from build123d import *

# Parameters (mm, degrees)
BOSS_EXTRUDE1_DEPTH = 8
FILLET1_R           = 0.5
FILLET2_R           = 0.25


with BuildPart() as part:
    # Sketch1 → Boss-Extrude1 (new body)
    with BuildSketch(Plane.XY):
        Polygon((14, 0), (-14, 0), (-14, 7), (-7, 10), (7, 10), (14, 7), align=None)
        Polygon((12.5, 1.5), (-12.5, 1.5), (-12.5, 6.010905763), (-6.692113447, 8.5), (6.692113447, 8.5), (12.5, 6.010905763), align=None, mode=Mode.SUBTRACT)
    extrude(amount=BOSS_EXTRUDE1_DEPTH)

    # Fillet1
    fillet1_edges = [part.edges().sort_by_distance(p)[0] for p in [
        (14, 0, 4),
        (-14, 0, 4),
        (-14, 7, 4),
        (-7, 10, 4),
        (7, 10, 4),
        (14, 7, 4),
        (12.5, 1.5, 4),
        (12.5, 6.010905763, 4),
        (6.692113447, 8.5, 4),
        (-6.692113447, 8.5, 4),
        (-12.5, 6.010905763, 4),
        (-12.5, 1.5, 4),
    ]]
    fillet(fillet1_edges, radius=FILLET1_R)

    # Fillet2
    fillet2_edges = [part.edges().sort_by_distance(p)[0] for p in [
        (0, 1.5, 0),
        (0, 1.5, 8),
        (12.5, 3.840603842, 0),
        (12.5, 3.840603842, 8),
        (9.491701947, 7.300176357, 0),
        (9.491701947, 7.300176357, 8),
        (0, 8.5, 0),
        (0, 8.5, 8),
        (-9.491701947, 7.300176357, 0),
        (-9.491701947, 7.300176357, 8),
        (-12.5, 3.840603842, 0),
        (-12.5, 3.840603842, 8),
        (10.395645224, 8.544723476, 0),
        (10.395645224, 8.544723476, 8),
        (14, 3.585150961, 0),
        (0, 0, 0),
        (-14, 3.585150961, 0),
        (-10.395645224, 8.544723476, 0),
        (0, 10, 0),
        (6.997904085, 9.989788861, 0),
        (-6.997904085, 9.989788861, 0),
        (-13.917420546, 6.945547425, 0),
        (-13.853553391, 0.146446609, 0),
        (13.853553391, 0.146446609, 0),
        (13.917420546, 6.945547425, 0),
        (14, 3.585150961, 8),
        (0, 10, 8),
        (-10.395645224, 8.544723476, 8),
        (-14, 3.585150961, 8),
        (0, 0, 8),
        (6.997904085, 9.989788861, 8),
        (-6.997904085, 9.989788861, 8),
        (-13.917420546, 6.945547425, 8),
        (-13.853553391, 0.146446609, 8),
        (13.853553391, 0.146446609, 8),
        (13.917420546, 6.945547425, 8),
        (12.353553391, 1.646446609, 0),
        (12.353553391, 1.646446609, 8),
        (12.417420546, 5.956453188, 0),
        (12.417420546, 5.956453188, 8),
        (6.690017532, 8.489788861, 0),
        (6.690017532, 8.489788861, 8),
        (-6.690017532, 8.489788861, 0),
        (-6.690017532, 8.489788861, 8),
        (-12.417420546, 5.956453188, 0),
        (-12.417420546, 5.956453188, 8),
        (-12.353553391, 1.646446609, 0),
        (-12.353553391, 1.646446609, 8),
    ]]
    fillet(fillet2_edges, radius=FILLET2_R)


solid = part.part
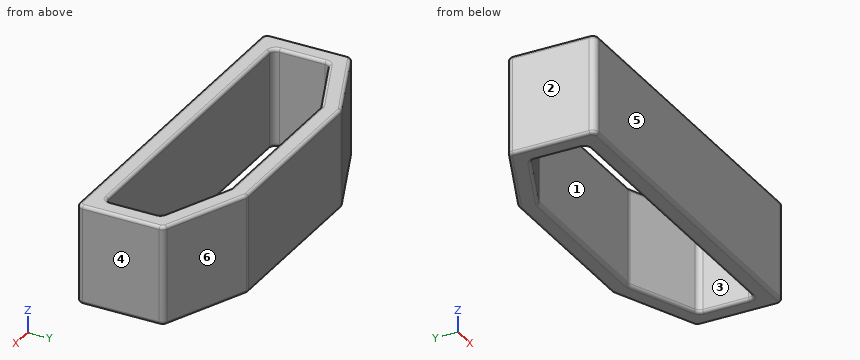
Geometry check sheet. Reference: the model listing, model coordinates, mm. Face numbers are marked on the shaded views. A direction names the side the tool comes from. Round coordinates to 2 decimals unless told otherwise and drop trailing zeros. Order: outer loops, then holes, each group sorted by start corner. A loop starts at its lowest first (then second) coordinate and runs counter-clockwise, first axis right, second up. Notation, with made-up numbers: M 75.25,12 L 85.25,12 A25 cw 85.25,35 Z; hole C -23.5,-20 d7. An arc over 180 degrees is marked long. Write each question's results on one line, items separated by ' | '. Start each with the question number.
1. Go/stop test with a flat-tipped pin: P1, Ø1.5, axis at x = -6.5, y = 7.5, coming from the +Z side. Record where the tip stops, or that it passes through.
2. Draft check along Y on the marked faces 3, 4, 5 and 6. Enter one of: pulls with the +Y half, pulls with the -Y half, needs draft (parallel to the pull), parting line crosses it, or undercut.
3. Set-up check for the marked faces 1 and 2: record each of +Z, -Z, +X, -X, +Y, -Y from which the full face is reachable in a straight line by a thin tool's end or side.
4. Cross-section at B-B on z = 6.75. Record the boundary of the cut face in (x, y), plus the area to 3 significant figures.
5. Material ranges on L1, parallel to X at y = 5.75, z = 4.25; L2, parallel to Y at x = -2.5, z = 4; L3, parallel to Y at x = -10, z = 6.5, recorded low to high. Write a range as from..to.
6. Cross-section at A-A on y = 4.5. Record the boundary of the cut face in (x, z), plus the area to 3 significant figures.
7. Cross-section at C-C on x = -1.75. Record the boundary of the cut face in (y, z), plus the area to 3 significant figures.
Resolved:
1) P1: through
2) face 3: undercut | face 4: needs draft | face 5: pulls with the -Y half | face 6: pulls with the +Y half
3) face 1: +Z, -Z | face 2: +Z, -Z, -X, +Y, -Y
4) outline: M -14,0.5 A0.5 ccw -13.5,0 L 13.5,0 A0.5 ccw 14,0.5 L 14,6.67 A0.5 ccw 13.7,7.13 L 7.09,9.96 A0.5 ccw 6.9,10 L -6.9,10 A0.5 ccw -7.09,9.96 L -13.7,7.13 A0.5 ccw -14,6.67 Z; hole M -12.5,2 A0.5 ccw -12,1.5 L 12,1.5 A0.5 ccw 12.5,2 L 12.5,5.68 A0.5 ccw 12.2,6.14 L 6.79,8.46 A0.5 ccw 6.59,8.5 L -6.59,8.5 A0.5 ccw -6.79,8.46 L -12.2,6.14 A0.5 ccw -12.5,5.68 Z | area: 98.5 mm2
5) L1: -14..-12.5, 12.5..14 | L2: 0..1.5, 8.5..10 | L3: 0..1.5, 7.08..8.71
6) outline: M -14,0.25 A0.25 ccw -13.75,0 L -12.75,0 A0.25 ccw -12.5,0.25 L -12.5,7.75 A0.25 ccw -12.75,8 L -13.75,8 A0.25 ccw -14,7.75 Z; M 12.5,0.25 A0.25 ccw 12.75,0 L 13.75,0 A0.25 ccw 14,0.25 L 14,7.75 A0.25 ccw 13.75,8 L 12.75,8 A0.25 ccw 12.5,7.75 Z | area: 23.9 mm2
7) outline: M 0,0.25 A0.25 ccw 0.25,0 L 1.25,0 A0.25 ccw 1.5,0.25 L 1.5,7.75 A0.25 ccw 1.25,8 L 0.25,8 A0.25 ccw 0,7.75 Z; M 8.5,0.25 A0.25 ccw 8.75,0 L 9.75,0 A0.25 ccw 10,0.25 L 10,7.75 A0.25 ccw 9.75,8 L 8.75,8 A0.25 ccw 8.5,7.75 Z | area: 23.9 mm2
